from build123d import *
from build123d.topology import SkipClean

# Parameters (mm, degrees)
SKETCH_1_R               = 23
SKETCH_1_R_2             = 9.25
EXTRUDE_1_DEPTH          = 3
EXTRUDE_START            = 6
EXTRUDE_2_DEPTH          = 6
SKETCH_3_R               = 1.6
CUT_EXTRUDE_1_DEPTH      = 40.862262856
FILLET_3_R               = 0.5
SKETCH_4_R               = 25
SKETCH_4_R_2             = 23
CUT_EXTRUDE_2_DEPTH      = 10
SKETCH_5_R               = 25
SKETCH_5_R_2             = 9.25
EXTRUDE_3_DEPTH          = 3
PATTERN_CIRCULAR_1_COUNT = 3
SKETCH_12_R              = 3
SKETCH_12_R_2            = 1.55
EXTRUDE_4_DEPTH          = 2
HOLE_WIZARD_M3_1_D       = 2.5
HOLE_WIZARD_M3_1_DEPTH   = 12.5
HOLE_WIZARD_M3_1_TIP     = 0.751075774
SKETCH_16_R              = 3
SKETCH_16_R_2            = 1.55
EXTRUDE_5_DEPTH          = 3


with BuildPart() as part:
    # 草图1 → 凸台-拉伸1 (new body)
    with BuildSketch(Plane.XY):
        Circle(SKETCH_1_R)
        Circle(SKETCH_1_R_2, mode=Mode.SUBTRACT)
    extrude(amount=EXTRUDE_1_DEPTH)

    # 草图2 → 凸台-拉伸2 (add)
    with BuildSketch(Plane(origin=(0, 0, 0), x_dir=(-1, 0, 0), z_dir=(0, 0, -1)).offset(EXTRUDE_START)):
        with BuildLine():
            Line((22, 9), (2.136000936, 9))
            ThreePointArc((2.136000936, 9), (6.215002341, 6.851003277), (8.75, 3))
            Line((8.75, 3), (22, 3))
            Line((22, 3), (22, 9))
        make_face()
        with BuildLine():
            Line((-22, 9), (-22, 3))
            Line((-22, 3), (-8.75, 3))
            ThreePointArc((-8.75, 3), (-6.215002341, 6.851003277), (-2.136000936, 9))
            Line((-2.136000936, 9), (-22, 9))
        make_face()
        with BuildLine():
            Line((22, -3), (8.75, -3))
            ThreePointArc((8.75, -3), (6.215002341, -6.851003277), (2.136000936, -9))
            Line((2.136000936, -9), (22, -9))
            Line((22, -9), (22, -3))
        make_face()
        with BuildLine():
            Line((-22, -9), (-2.136000936, -9))
            ThreePointArc((-2.136000936, -9), (-6.215002341, -6.851003277), (-8.75, -3))
            Line((-8.75, -3), (-22, -3))
            Line((-22, -3), (-22, -9))
        make_face()
    extrude(amount=-EXTRUDE_2_DEPTH)

    # 草图3 → 切除-拉伸1 (cut, through all)
    with BuildSketch(Plane.XZ.offset(9)):
        with Locations(Location((-17.5, -3, 0), (0, 0, 270))):
            Circle(SKETCH_3_R)
        with Locations(Location((17.5, -3, 0), (0, 0, 270))):
            Circle(SKETCH_3_R)
    extrude(amount=-CUT_EXTRUDE_1_DEPTH, mode=Mode.SUBTRACT)

    # 圆角3
    # the kernel refuses this fillet: 0.5 mm, written as the material it takes off along each edge
    with BuildSketch(Plane(origin=(2.136000936, 9, -12.600605893), x_dir=(0.9314269408293101, -0.36392836368899956, 0), z_dir=(0, 0, 1))) as fillet_3_piece_1:
        with BuildLine():
            CenterArc((2.641157044, 0.49514561), FILLET_3_R, 111.34164725, 150.667889832)
            Line((2.459192862, 0.960859081), (0, 0))
            ThreePointArc((0, 0), (1.285826456, 0.089806207), (2.571652911, 0))
        make_face()
    extrude(amount=12.600605893, mode=Mode.SUBTRACT)
    with BuildSketch(Plane(origin=(-2.136000936, 9, -12.600605893), x_dir=(-0.931426940829308, -0.3639283636890051, 0), z_dir=(0, 0, 1))) as fillet_3_piece_2:
        with BuildLine():
            CenterArc((2.641157044, -0.49514561), FILLET_3_R, 97.990462918, 150.667889832)
            Line((2.459192862, -0.960859081), (0, 0))
            ThreePointArc((0, 0), (1.285826456, -0.089806207), (2.571652911, 0))
        make_face()
    extrude(amount=12.600605893, mode=Mode.SUBTRACT)
    with BuildSketch(Plane(origin=(-2.136000936, -9, -12.600605893), x_dir=(-1, 0, 0), z_dir=(0, 0, 1))) as fillet_3_piece_3:
        with BuildLine():
            CenterArc((2.640242357, -0.5), FILLET_3_R, 90, 150.667889832)
            ThreePointArc((2.395306804, -0.935897436), (1.230336428, -0.384300797), (0, 0))
            Line((0, 0), (2.640242357, 0))
        make_face()
    extrude(amount=12.600605893, mode=Mode.SUBTRACT)
    with BuildSketch(Plane(origin=(2.136000936, -9, -12.600605893), x_dir=(1, 0, 0), z_dir=(0, 0, 1))) as fillet_3_piece_4:
        with BuildLine():
            CenterArc((2.640242357, 0.5), FILLET_3_R, 119.332110168, 150.667889832)
            ThreePointArc((2.395306804, 0.935897436), (1.230336428, 0.384300797), (0, 0))
            Line((0, 0), (2.640242357, 0))
        make_face()
    extrude(amount=12.600605893, mode=Mode.SUBTRACT)

    # 草图4 → 切除-拉伸2 (cut)
    with SkipClean():  # the faces are left unmerged after this step: merging them gives an invalid solid
        with BuildSketch(Plane(origin=(0, 0, -6), x_dir=(-1, 0, 0), z_dir=(0, 0, -1))):
            Circle(SKETCH_4_R)
            with Locations(Location((0, 0, 0), (0, 0, 16.957426294))):
                Circle(SKETCH_4_R_2, mode=Mode.SUBTRACT)
        extrude(amount=-CUT_EXTRUDE_2_DEPTH, mode=Mode.SUBTRACT)
    add(part.part.scale(1), mode=Mode.REPLACE)  # the faces are merged on a copy

    # 草图5 → 凸台-拉伸3 (add)
    with SkipClean():  # the faces are left unmerged after this step: merging them gives an invalid solid
        with BuildSketch(Plane.XY):
            Circle(SKETCH_5_R)
            with Locations(Location((0, 0, 0), (0, 0, 198.924644416))):
                Circle(SKETCH_5_R_2, mode=Mode.SUBTRACT)
        extrude(amount=EXTRUDE_3_DEPTH)
    add(part.part.scale(1), mode=Mode.REPLACE)  # the faces are merged on a copy

    # 草图11 → 切除-旋转1 (revolve, cut)
    with BuildSketch(Plane(origin=(0, 0, 0), x_dir=(1, 0, 0), z_dir=(0, 1, 0))):
        Polygon((21.55, -3), (21.55, -1.45), (23, 0), (20, 0), (20, -3), align=None)
    cut_revolve_1 = revolve(axis=Axis((20, 0, 8.062210134), (0, 0, -1)), mode=Mode.SUBTRACT)

    # 阵列(圆周)1: 切除-旋转1 ×3 about axis
    pattern_circular_1_axis = Axis((0, 0, 0), (0, 0, 1))
    for i in range(1, PATTERN_CIRCULAR_1_COUNT):
        add(cut_revolve_1.rotate(pattern_circular_1_axis, i * 360 / PATTERN_CIRCULAR_1_COUNT), mode=Mode.SUBTRACT)

    # 草图12 → 凸台-拉伸4 (add)
    # profile 1 of 2: a face of its own
    with BuildSketch(Plane(origin=(0, 0, 0), x_dir=(-1, 0, 0), z_dir=(0, 0, -1))):
        with Locations((10, 17.320508076)):
            Circle(SKETCH_12_R)
        with Locations(Location((10, 17.320508076, 0), (0, 0, 60))):
            Circle(SKETCH_12_R_2, mode=Mode.SUBTRACT)
    # profile 2 of 2: a face of its own
    with BuildSketch(Plane(origin=(0, 0, 0), x_dir=(-1, 0, 0), z_dir=(0, 0, -1))):
        with Locations((10, -17.320508076)):
            Circle(SKETCH_12_R)
        with Locations(Location((10, -17.320508076, 0), (0, 0, 300))):
            Circle(SKETCH_12_R_2, mode=Mode.SUBTRACT)
    extrude(amount=-EXTRUDE_4_DEPTH)

    # M3 螺纹孔1
    with Locations(Plane(origin=(0, 0, 0), x_dir=(-1, 0, 0), z_dir=(0, 0, -1))):
        with Locations((-10, 17.320508076), (-10, -17.320508076)):
            Hole(HOLE_WIZARD_M3_1_D / 2, depth=HOLE_WIZARD_M3_1_DEPTH)
            with Locations((0, 0, -(HOLE_WIZARD_M3_1_DEPTH + HOLE_WIZARD_M3_1_TIP / 2))):  # 118° drill point
                Cone(0, HOLE_WIZARD_M3_1_D / 2, HOLE_WIZARD_M3_1_TIP, mode=Mode.SUBTRACT)

    # 草图16 → 凸台-拉伸5 (add)
    with BuildSketch(Plane(origin=(0, 0, 0), x_dir=(-1, 0, 0), z_dir=(0, 0, -1))):
        with Locations((-20, 0)):
            Circle(SKETCH_16_R)
        with Locations(Location((-20, 0, 0), (0, 0, 180))):
            Circle(SKETCH_16_R_2, mode=Mode.SUBTRACT)
    extrude(amount=-EXTRUDE_5_DEPTH)


solid = part.part
Model file for the job. Use its own axes, mm. A direction names the side the tool comes from. Give positions to 0.01 mm unless a question says otherwise; leave off trailing zeros. Order: outer loops, then holes, each group sorted by start corner. A loop starts at its lowest first (then second) coordinate and runs counter-clockwise, first axis right, second up. Notation, with made-up numbers: (20, 83.5) -> (67, 83.5) arc R16 ccw to (67, 113.5) -> close; hole circle Ø9 at (36.25, 71.5). An arc over 180 degrees is marked (long way). Use CSV: the item, a comma, the result in double quotes.
1. 3-axis set-ups, long thin cutter, end or side, ignore diameter. For faces 5 (the cylindrical face through (21.6, 7.9, -3)), 6 (the flat face through (-15, 3, -3)), 7 (the cylindrical face through (-21.62, 7.85, -3.04)): which of +Z, -Z, +X, -X, +Y, -Y reach the whole face in a straight line?
Outcome:
face 5,"-Z, +X, +Y"
face 6,"-Z, +X, -X"
face 7,"-Z, -X, +Y"
2. Drop flat-ended pins along their axis: pin 1 (3 mm diameter, centred on x = 14, z = -4, fed in from +Y); pin 2 (1.1 mm diameter, centred on y = 4, z = -2, fed in from -X); pin 3 (3 mm diameter, centred on x = 17.5, z = -2.5, fed in from -Y). Give the stop position or say it passes through.
Outcome:
pin 1,"y = 9"
pin 2,"x = -22"
pin 3,"y = -9"
3. Band-saw the part on B-B, the plane y = -5. Give the cut face in (x, z), then the cut area to 3 significant figures.
Outcome:
outline,"(-24.49, 0) -> (-22, 0) -> (-22, -6) -> (-7.78, -6) -> (-7.78, 3) -> (-24.49, 3) -> close; (7.78, -6) -> (22, -6) -> (22, 0) -> (24.49, 0) -> (24.49, 3) -> (7.78, 3) -> close; hole circle Ø3.2 at (-17.5, -3); hole circle Ø3.2 at (17.5, -3)"
area,"255 mm²"
4. Drill centre lines: line 1 along Y through (x, z) = (-9, -3.5); line 2 along X through (y, z) = (8, -2); line 3 along X through (y, z) = (7.3, -3). Where is each one in solid material? Low to high. Write a range as from..to.
Outcome:
line 1,"-9..-3, 3..9"
line 2,"-21.56..-18.75, -16.25..-4.64, 4.64..16.25, 18.75..21.56"
line 3,"-21.81..-19.1, -15.9..-5.68, 5.68..15.9, 19.1..21.81"
5. Mould opens along X. For faces 1 (the flat face through (-15, -3, -3)), 2 (the cylindrical face through (21.478, -0.466, 1.479)), 3 (the cylindrical face through (23.846, 7.509, 1.479)), 4 (the cylindrical face through (-10.336, 18.834, 1.479)) say: +X half, -X half, draft (parallel to the pull), parting line (faces both ways), or undercut.
Outcome:
face 1,"draft"
face 2,"undercut"
face 3,"parting line"
face 4,"undercut"
6. Band-saw the part on D-D, the plane z = -3. Count the separate pieces of the cut face and the enclosed holes in it, then the cut area to 3 significant figures.
Outcome:
separate pieces,"8"
enclosed holes,"0"
area,"286 mm²"
7. Band-saw the part on A-A, the plane x = 20. Give the cut face in (y, z), then the cut area to 3 significant figures.
Outcome:
outline,"(-15, 0) -> (-9, 0) -> (-9, -6) -> (-3, -6) -> (-3, 0) -> (-1.55, 0) -> (-1.55, 3) -> (-15, 3) -> close; (1.55, 0) -> (3, 0) -> (3, -6) -> (9, -6) -> (9, 0) -> (15, 0) -> (15, 3) -> (1.55, 3) -> close"
area,"153 mm²"
8. Band-saw the part on C-C, the plane x = -17.5. Give the cut face in (y, z).
Outcome:
outline,"(-17.85, 0) -> (-9, 0) -> (-9, -1.4) -> (-3, -1.4) -> (-3, 0) -> (3, 0) -> (3, -1.4) -> (9, -1.4) -> (9, 0) -> (17.85, 0) -> (17.85, 3) -> (-17.85, 3) -> close; (-9, -6) -> (-3, -6) -> (-3, -4.6) -> (-9, -4.6) -> close; (3, -6) -> (9, -6) -> (9, -4.6) -> (3, -4.6) -> close"
